from build123d import *

# Parameters (mm, degrees)
SKETCH_1_W          = 566.5
SKETCH_1_H          = 95
EXTRUDE_1_DEPTH     = 3
SKETCH_2_W          = 566.5
SKETCH_2_H          = 3
EXTRUDE_2_DEPTH     = 17
SKETCH_3_R          = 3.5
CUT_EXTRUDE_1_DEPTH = 575.661857095
SKETCH_4_R          = 2.5
CUT_EXTRUDE_2_DEPTH = 575.270189023
FILLET_1_R          = 5
FILLET_2_R          = 2


with BuildPart() as part:
    # 스케치1 → 보스-돌출1 (new body)
    with BuildSketch(Plane.XY):
        with Locations((283.25, 47.5)):
            Rectangle(SKETCH_1_W, SKETCH_1_H)
    extrude(amount=EXTRUDE_1_DEPTH)

    # 스케치2 → 보스-돌출2 (add)
    with BuildSketch(Plane.XY.offset(3)):
        with Locations((283.25, 1.5)):
            Rectangle(SKETCH_2_W, SKETCH_2_H)
    extrude(amount=EXTRUDE_2_DEPTH)

    # 스케치3 → 컷-돌출1 (cut, through all)
    with BuildSketch(Plane.XY.offset(3)):
        with Locations((53.25, 55)):
            Circle(SKETCH_3_R)
        with Locations((53.25, 20)):
            Circle(SKETCH_3_R)
        with Locations((283.25, 55)):
            Circle(SKETCH_3_R)
        with Locations((283.25, 20)):
            Circle(SKETCH_3_R)
        with Locations((513.25, 55)):
            Circle(SKETCH_3_R)
        with Locations((513.25, 20)):
            Circle(SKETCH_3_R)
    extrude(amount=-CUT_EXTRUDE_1_DEPTH, mode=Mode.SUBTRACT)

    # 스케치4 → 컷-돌출2 (cut, through all)
    with BuildSketch(Plane(origin=(0, 3, 0), x_dir=(1, 0, 0), z_dir=(0, 1, 0))):
        with Locations(Location((60, -11.5, 0), (0, 0, 270))):
            Circle(SKETCH_4_R)
        with Locations(Location((506.5, -11.5, 0), (0, 0, 270))):
            Circle(SKETCH_4_R)
    extrude(amount=-CUT_EXTRUDE_2_DEPTH, mode=Mode.SUBTRACT)

    # 필렛1
    fillet_1_edges = [part.edges().sort_by_distance(p)[0] for p in [
        (283.25, 0, 0),
    ]]
    fillet(fillet_1_edges, radius=FILLET_1_R)

    # 필렛2
    fillet_2_edges = [part.edges().sort_by_distance(p)[0] for p in [
        (283.25, 3, 3),
    ]]
    fillet(fillet_2_edges, radius=FILLET_2_R)


solid = part.part
The model under review builds one solid part; all positions refer to its coordinate system, in mm. A direction names the side the tool comes from. Coordinates: 2 decimals unless noted, no trailing zeros. Loops run counter-clockwise (first coordinate to the right, second up) from the corner with the lowest first, then second, coordinate; pieces in that order, holes last. Notation, with made-up numbers: (8, 16) -> (30, 16) arc R12 ccw to (30, 29) -> close; hole circle Ø2 at (2, 57.25). An arc over 180 degrees is marked (long way). Use a Markdown table: item, result. Add a question column.
1. Clearance check with flat-ended pins moving along their axes: pin 1 Ø12 at (x, z) = (416, 13.5) entering from +Y; pin 2 Ø1 at (x, z) = (349.5, 2) entering from -Y; pin 3 Ø4 at (x, y) = (141.5, 55.5) entering from +Z. State where each tip first meets the part, or that it passes through.
2. To check wall thickness, follow line 1 (Y direction, x = 283.25, z = 1.3); line 2 (Y direction, x = 283.25, z = 0.75); line 3 (Y direction, x = 458, z = 4.5). State the ranges of each line that lie inside material, in increasing order.
3. Add section A-A on y = 43.5. Write out the cut boundary in (x, z).
4. Machinability: for faces 1 (the face through (279, 3, 12)), 2 (the face through (0, 40, 2)), which of the approach directions +Z, -Z, +X, -X, +Y, -Y give a long, thin tool a straight path to every point of the face, cutting with its end or side? Answer none if there is none.
Returned:
| question | item | result |
|---|---|---|
| 1 | pin 1 | stops at y = 3 |
| 1 | pin 2 | stops at y = 0.67 |
| 1 | pin 3 | stops at z = 3 |
| 2 | line 1 | y = 1.64 to 16.5, 23.5 to 51.5, 58.5 to 95 |
| 2 | line 2 | y = 2.37 to 16.5, 23.5 to 51.5, 58.5 to 95 |
| 2 | line 3 | y = 0.03 to 3.06 |
| 3 | outline | (0, 0) -> (566.5, 0) -> (566.5, 3) -> (0, 3) -> close |
| 4 | face 1 | +Z, +X, -X, +Y |
| 4 | face 2 | +Z, -Z, -X, +Y, -Y |
